```python
from build123d import *

# Parameters (mm, degrees)
BOSS_EXTRUDE1_DEPTH       = 16.51
CUT_EXTRUDE1_REACH        = 14.446
SKETCH2_W                 = 3.96875
SKETCH2_H                 = 20.828
F_6_32_TAPPED_HOLE1_D     = 2.7051
F_6_32_TAPPED_HOLE1_DEPTH = 3.96875
F_6_32_TAPPED_HOLE2_D     = 2.7051
F_6_32_TAPPED_HOLE2_DEPTH = 3.175


with BuildPart() as part:
    # Sketch1 → Boss-Extrude1 (new body, symmetric)
    with BuildSketch(Plane.XY):
        Polygon((0, 12.446), (0, 0), (7.9375, 0), (7.9375, 3.175), (3.96875, 3.175), (3.96875, 12.446), align=None)
    extrude(amount=BOSS_EXTRUDE1_DEPTH, both=True)

    # Sketch2 → Cut-Extrude1 (cut, up to next)
    with BuildSketch(Plane(origin=(0, 12.446, 0), x_dir=(1, 0, 0), z_dir=(0, 1, 0)), mode=Mode.PRIVATE) as cut_extrude1_sk1:
        with Locations((1.984375, 0)):
            Rectangle(SKETCH2_W, SKETCH2_H)
    cut_extrude1_tool1 = extrude(cut_extrude1_sk1.sketch, amount=-CUT_EXTRUDE1_REACH, mode=Mode.PRIVATE) & part.part
    add(cut_extrude1_tool1.solids().sort_by_distance((1.984375, 12.446, 0))[0], mode=Mode.SUBTRACT)

    # #6-32 Tapped Hole1
    with Locations(Plane(origin=(3.96875, 0, 0), x_dir=(0, 0, -1), z_dir=(1, 0, 0))):
        with Locations((-13.470384182, 9.525), (13.470384182, 9.525)):
            Hole(F_6_32_TAPPED_HOLE1_D / 2, depth=F_6_32_TAPPED_HOLE1_DEPTH)

    # #6-32 Tapped Hole2
    with Locations(Plane.XZ):
        with Locations((5.3975, 13.470384182), (5.3975, -13.470384182)):
            Hole(F_6_32_TAPPED_HOLE2_D / 2, depth=F_6_32_TAPPED_HOLE2_DEPTH)


solid = part.part
```
Check sheet for the modelled part. Datum: model origin and axes. Units: mm. A direction names the side the tool comes from. Give positions to 0.01 mm unless a question says otherwise; leave off trailing zeros. Order: outer loops, then holes, each group sorted by start corner. A loop starts at its lowest first (then second) coordinate and runs counter-clockwise, first axis right, second up. Notation, with made-up numbers: (82, -12) -> (102, -12) arc R24 ccw to (102, 19) -> close; hole circle Ø4 at (-12, 7). An arc over 180 degrees is marked (long way). Return JSON: item names as keys, results as strings.
1. Go/stop test with flat-tipped pins: P1, Ø1, axis at x = 5, z = 2, coming from the +Y side (3 decimals); P2, Ø3, axis at y = 10, z = 13.5, coming from the +X side; P3, Ø1.6, axis at y = 9.52, z = 13.47, coming from the +X side; P4, Ø3.5, axis at y = 2, z = -3.5, coming from the -X side. Record where each tip stops, or that it passes through.
From the geometry:
{"P1": "y = 3.175", "P2": "x = 3.97", "P3": "through", "P4": "x = 3.97"}
2. Cross-section at D-D, the plane x = 1.25. Record the cut outline in (y, z) (3 decimals), plus the area to 3 significant figures.
From the geometry:
{"outline": "(0, -16.51) -> (12.446, -16.51) -> (12.446, -10.414) -> (0, -10.414) -> close; (0, 10.414) -> (12.446, 10.414) -> (12.446, 16.51) -> (0, 16.51) -> close; hole circle Ø2.705 at (9.525, -13.47); hole circle Ø2.705 at (9.525, 13.47)", "area": "140 mm^2"}
3. Cross-section at A-A, the plane y = 7.5. Record the cut outline in (x, z), plus the area to 3 significant figures.
From the geometry:
{"outline": "(0, -16.51) -> (3.97, -16.51) -> (3.97, -10.41) -> (0, -10.41) -> close; (0, 10.41) -> (3.97, 10.41) -> (3.97, 16.51) -> (0, 16.51) -> close", "area": "48.4 mm^2"}
4. Cross-section at C-C, the plane y = 9. Record the cut outline in (x, z).
From the geometry:
{"outline": "(0, -16.51) -> (3.97, -16.51) -> (3.97, -14.72) -> (0, -14.72) -> close; (0, -12.22) -> (3.97, -12.22) -> (3.97, -10.41) -> (0, -10.41) -> close; (0, 10.41) -> (3.97, 10.41) -> (3.97, 12.22) -> (0, 12.22) -> close; (0, 14.72) -> (3.97, 14.72) -> (3.97, 16.51) -> (0, 16.51) -> close"}
5. Material ranges on probe 1 along Z at (x, y) = (2, 9.5); probe 2 along Z at (x, y) = (1.5, 4.75); probe 3 along Z at (x, y) = (2, 10.25), recorded low to high. Write a range as [from, to].
From the geometry:
{"probe 1": "[-16.51, -14.82], [-12.12, -10.41], [10.41, 12.12], [14.82, 16.51]", "probe 2": "[-16.51, -10.41], [10.41, 16.51]", "probe 3": "[-16.51, -14.61], [-12.33, -10.41], [10.41, 12.33], [14.61, 16.51]"}
6. Set-up check for faces 1 (the flat face through (0, 6, 14)), 2 (the flat face through (3.969, 2, 0)), 3 (the flat face through (3.969, 8, 14)): record each of +Z, -Z, +X, -X, +Y, -Y from which the full face is reachable in a straight line by a thin tool's end or side.
From the geometry:
{"face 1": "+Z, -Z, -X, +Y, -Y", "face 2": "-X, +Y, -Y", "face 3": "+Z, -Z, +X, +Y"}
7. Mould release check, pull along Z, two halves, no side actions. Record for faces 4 (the flat face through (2, 12.446, 14)), 5 (the cylindrical face through (1.957, 10.866, 13.294)), 6 (the flat face through (3, 5, -16.51)), 7 (the flat face through (2, 6, -10.414)): +Z half, -Z half, draft (parallel to the pull), parting line (faces both ways), or undercut.
From the geometry:
{"face 4": "draft", "face 5": "undercut", "face 6": "-Z half", "face 7": "undercut"}
8. Cross-section at B-B, the plane x = 5.25. Record the cut outline in (y, z) (3 decimals).
From the geometry:
{"outline": "(0, -16.51) -> (3.175, -16.51) -> (3.175, -14.815) -> (0, -14.815) -> close; (0, -12.126) -> (3.175, -12.126) -> (3.175, 12.126) -> (0, 12.126) -> close; (0, 14.815) -> (3.175, 14.815) -> (3.175, 16.51) -> (0, 16.51) -> close"}
